Work out the finished part from the listing and answer in its coordinate system (mm). A direction names the side the tool comes from. Round coordinates to 2 decimals unless told otherwise and drop trailing zeros. Loops run counter-clockwise (first coordinate to the right, second up) from the corner with the lowest first, then second, coordinate; pieces in that order, holes last.
from build123d import *

# Parameters (mm, degrees)
F0_W      = 17.3620246351
F0_H      = 23.728100583
F1_DEPTH  = 1.27
F3_DEPTH  = 113.6904
F4_W      = 79.9476280808
F4_H      = 47.4562011659
F5_DEPTH  = 1.4986
F7_DEPTH  = 79.9338
F8_DEPTH  = 39.878
F10_DEPTH = 17.018
F12_DEPTH = 16.8402
F13_R     = 6.5036466471
F14_DEPTH = 198.628
F15_R     = 7.9715135089
F16_DEPTH = 343.916


with BuildPart() as f1:
    # F0 (on Top) → F1 (new body)
    with BuildSketch(Plane.XY):
        with Locations((-48.1796208769, 11.8640502915)):
            Rectangle(F0_W, F0_H)
        with Locations((-48.1796208769, -11.8640502915)):
            Rectangle(F0_W, F0_H)
        Polygon((39.4986085594, 0), (39.4986085594, 23.728100583), (-39.4986085594, 23.728100583), (-39.4986085594, 0), (-39.4986085594, -23.728100583), (39.4986085594, -23.728100583), align=None)
        with Locations((48.1796208769, 11.8640502915)):
            Rectangle(F0_W, F0_H)
        with Locations((48.1796208769, -11.8640502915)):
            Rectangle(F0_W, F0_H)
    extrude(amount=-F1_DEPTH)

    # F2 (on face) → F3 (join)
    with BuildSketch(Plane(origin=(-56.8606331944, 0, 0), x_dir=(0, -1, 0), z_dir=(-1, 0, 0))):
        with BuildLine():
            Line((23.728100583, -1.27), (-23.728100583, -1.27))
            ThreePointArc((-23.728100583, -1.27), (0, -24.998100583), (23.728100583, -1.27))
        make_face()
    extrude(amount=-F3_DEPTH)

    # F4 (on face) → F5 (join)
    with BuildSketch(Plane.XY):
        Rectangle(F4_W, F4_H)
    extrude(amount=F5_DEPTH)

    # F6 (on face) → F7 (join)
    with BuildSketch(Plane(origin=(-39.9738140404, 0, 0), x_dir=(0, -1, 0), z_dir=(-1, 0, 0))):
        with BuildLine():
            Line((-23.728100583, 1.4986), (23.728100583, 1.4986))
            ThreePointArc((23.728100583, 1.4986), (0, 25.226700583), (-23.728100583, 1.4986))
        make_face()
    extrude(amount=-F7_DEPTH)

    # F8 (add): faces of the model
    f8_faces = [f1.faces().sort_by_distance(p)[0] for p in [
        (-48.4172236174, 0, 0),
        (48.4172236174, 0, 0),
    ]]
    extrude(f8_faces, amount=F8_DEPTH)

    # F9 (on face) → F10 (join)
    with BuildSketch(Plane(origin=(-56.8606331944, 0, 0), x_dir=(0, -1, 0), z_dir=(-1, 0, 0))):
        with BuildLine():
            Line((-23.728100583, 39.878), (23.728100583, 39.878))
            ThreePointArc((23.728100583, 39.878), (0, 63.606100583), (-23.728100583, 39.878))
        make_face()
    extrude(amount=-F10_DEPTH)

    # F11 (on face) → F12 (join)
    with BuildSketch(Plane.YZ.offset(56.8606331944)):
        with BuildLine():
            Line((-23.728100583, 39.878), (23.728100583, 39.878))
            ThreePointArc((23.728100583, 39.878), (0, 63.606100583), (-23.728100583, 39.878))
        make_face()
    extrude(amount=-F12_DEPTH)

    # F13 (on face) → F14 (cut)
    with BuildSketch(Plane(origin=(-56.8606331944, 0, 0), x_dir=(0, -1, 0), z_dir=(-1, 0, 0))):
        with Locations((0, 39.878)):
            Circle(F13_R)
    extrude(amount=-F14_DEPTH, mode=Mode.SUBTRACT)

    # F15 (on face) → F16 (cut)
    with BuildSketch(Plane(origin=(-56.8606331944, 0, 0), x_dir=(0, -1, 0), z_dir=(-1, 0, 0))):
        Circle(F15_R)
    extrude(amount=-F16_DEPTH, mode=Mode.SUBTRACT)


solid = f1.part
Item 1: Section C-C, the plane x = -17 is taken. Give the vertices of the cut face in (y, z).
Item 2: Each of these flat-tipped pins is pushed along its axis until it touches: P1, Ø1, axis at y = 10, z = -2.5, coming from the +X side; P2, Ø11.5, axis at y = 0, z = 39.878, coming from the -X side; P3, Ø3, axis at x = -20.5, z = 24, coming from the -Y side; P4, Ø6, axis at x = -44, y = 8, coming from the +Z side. Where does it stop, or does it pass through?
Item 3: Straight lines are drawn through the part: line 1 (Z direction, x = -45.75, y = 0); line 2 (X direction, y = 17.5, z = 48.5); line 3 (Z direction, x = 11, y = 0). For each, find the intervals that lie inside material, in ascending order.
Item 4: Section B-B, the plane z = 0 is taken. Give the vertices of the cut face in (x, y).
Item 5: Determine the mould class of faces 4 (the face through (0, 23.728, -1)), 5 (the face through (56.83, 0, -13)), 6 (the face through (39.974, 5, 25)) for opening direction X: pulls with the +X half, pulls with the -X half, needs draft (parallel to the pull), parting line crosses it, or undercut.
Item 6: For faces 1 (the face through (-39.974, 0, 29)), 2 (the face through (-39.843, 0, 52)), 3 (the face through (-48.5, -0.5, 63.6)), determine the directions among +Z, -Z, +X, -X, +Y, -Y from which every point of the face is accessible in a straight line to the end or side of a thin tool.
Item 7: Section A-A, the plane y = 0 is taken. Give the vertices of the cut face in (x, z).
Answer below:
1. outline: (-23.73, -1.27) arc R23.73 ccw to (23.73, -1.27) - (23.73, 1.5) arc R23.73 ccw to (-23.73, 1.5) - close; hole circle Ø15.94 at (0, 0)
2. P1: stops at x = 56.83
2. P2: passes through
2. P3: stops at y = -11.04
2. P4: stops at z = 63.07
3. line 1: z = -25 to -7.97, 7.97 to 33.37, 46.38 to 63.61
3. line 2: x = -56.86 to -39.84, 40.02 to 56.86
3. line 3: z = -25 to -7.97, 7.97 to 25.23
4. outline: (-56.86, -23.73) - (56.86, -23.73) - (56.86, -7.97) - (-56.86, -7.97) - close; (-56.86, 7.97) - (56.86, 7.97) - (56.86, 23.73) - (-56.86, 23.73) - close
5. face 4: needs draft
5. face 5: pulls with the +X half
5. face 6: undercut
6. face 1: none
6. face 2: +Z, +Y, -Y
6. face 3: +Z, +X, -X
7. outline: (-56.86, -25) - (56.83, -25) - (56.83, -7.97) - (-56.86, -7.97) - close; (-56.86, 7.97) - (39.96, 7.97) - (39.96, 25.23) - (-39.97, 25.23) - (-39.97, 33.37) - (-56.86, 33.37) - close; (-56.86, 46.38) - (-39.84, 46.38) - (-39.84, 63.61) - (-56.86, 63.61) - close; (39.97, 7.97) - (56.86, 7.97) - (56.86, 33.37) - (39.97, 33.37) - close; (40.02, 46.38) - (56.86, 46.38) - (56.86, 63.61) - (40.02, 63.61) - close
